Work out the finished part from the listing and answer in its coordinate system (mm). Coordinates: 2 decimals unless noted, no trailing zeros. Write each loop counter-clockwise with the first axis right and the second up, starting at its lowest first coordinate (ties: lowest second). Pieces come first, ordered by that corner, then holes. Notation, with made-up numbers: (43, 16.5) - (91, 16.5) arc R22 ccw to (91, 30.5) - close; hole circle Ø9 at (71.25, 89). An arc over 180 degrees is marked (long way). Answer as a JSON object with one key per item and string values. Group by question number.
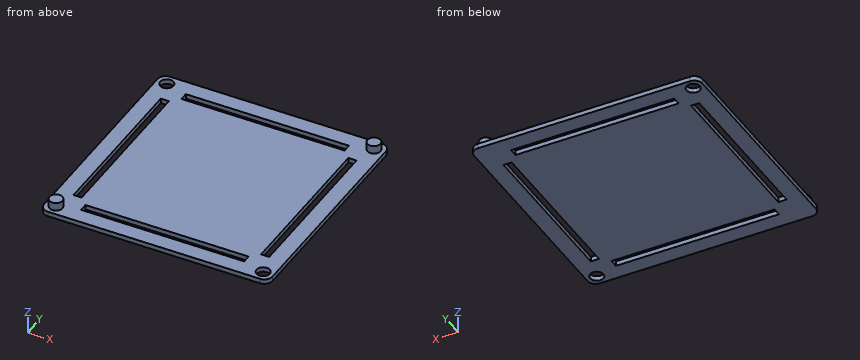
Autodesk Inventor part; units mm, degrees
ref_plane "YZ Plane" through (0, 0, 0) normal (1, 0, 0) x (0, 1, 0)
ref_plane "XZ Plane" through (0, 0, 0) normal (0, 1, 0) x (-1, 0, 0)
ref_plane "XY Plane" through (0, 0, 0) normal (0, 0, 1) x (1, 0, 0)
sketch "Sketch1" plane through (0, 0, 0) normal (0, 0, 1) x (1, 0, 0)
  line L0 (0, 0) -> (140, 0)
  line L1 (140, 0) -> (140, 140)
  line L2 (140, 140) -> (0, 140)
  line L3 (0, 140) -> (0, 0)
  dimension "d0" = 140
  dimension "d1" = 140
extrude "Extrusion1" add sketch "Sketch1" along normal blind 3
fillet "Fillet1" radius 5 4 edges at (140, 140, 1.5) (140, 0, 1.5) (0, 140, 1.5) (0, 0, 1.5)
sketch "Sketch4" plane through (0, 0, 3) normal (0, 0, 1) x (1, 0, 0)
  line L0 (135, 140) -> (5, 140)
  line L1 (0, 135) -> (0, 5)
  line L2 (140, 5) -> (140, 135)
  line L3 (5, 0) -> (135, 0)
  point P0 (0, 0)
  point P1 (6.5, 133.5)
  point P2 (133.5, 6.5)
  dimension "d30" = 6.5
  dimension "d31" = 6.5
  dimension "d34" = 6.5
  dimension "d35" = 6.5
hole "Hole2" at (133.5, 6.5, 3) at (6.5, 133.5, 3) direction (0, 0, -1) diameter 8.2 depth 15
sketch "Sketch5" plane through (0, 0, 3) normal (0, 0, 1) x (1, 0, 0)
  line L0 (20, 130) -> (120, 130)
  line L1 (120, 130) -> (120, 125)
  line L2 (120, 125) -> (20, 125)
  line L3 (20, 125) -> (20, 130)
  line L4 (135, 140) -> (5, 140)
  line L5 (140, 5) -> (140, 135)
  line L6 (20, 15) -> (120, 15)
  line L7 (120, 15) -> (120, 10)
  line L8 (120, 10) -> (20, 10)
  line L9 (20, 10) -> (20, 15)
  line L10 (5, 0) -> (135, 0)
  line L11 (10, 120) -> (15, 120)
  line L12 (15, 120) -> (15, 20)
  line L13 (15, 20) -> (10, 20)
  line L14 (10, 20) -> (10, 120)
  line L15 (0, 135) -> (0, 5)
  line L16 (125, 120) -> (130, 120)
  line L17 (130, 120) -> (130, 20)
  line L18 (130, 20) -> (125, 20)
  line L19 (125, 20) -> (125, 120)
  point P0 (0, 0)
  dimension "d45" = 10
  dimension "d46" = 5
  dimension "d47" = 20
  dimension "d48" = 100
  dimension "d49" = 100
  dimension "d50" = 5
  dimension "d51" = 20
  dimension "d52" = 10
  dimension "d53" = 5
  dimension "d54" = 100
  dimension "d55" = 20
  dimension "d56" = 10
  dimension "d57" = 5
  dimension "d58" = 100
  dimension "d59" = 10
  dimension "d60" = 20
extrude "Extrusion4" cut sketch "Sketch5" against normal blind 10
sketch "Sketch6" plane through (0, 0, 3) normal (0, 0, 1) x (1, 0, 0)
  circle A0 centre (6.5, 6.5) radius 4
  circle A1 centre (133.5, 133.5) radius 4
  line L0 (135, 140) -> (5, 140)
  line L1 (140, 5) -> (140, 135)
  line L2 (5, 0) -> (135, 0)
  line L3 (0, 135) -> (0, 5)
  point P0 (0, 0)
  dimension "d66" = 8
  dimension "d67" = 8
  dimension "d68" = 6.5
  dimension "d69" = 6.5
  dimension "d70" = 6.5
  dimension "d71" = 6.5
extrude "Extrusion5" add sketch "Sketch6" along normal blind 5
properties part number "Led deksel niet hub"
Q1. Section C-C on z = 5.5 is taken. Determine the outline of the cut face in (x, y).
Q2. Section D-D on y = 17 is taken. Determine the outline of the cut face in (x, z).
Q3. Section A-A on x = 53 is taken. Determine the outline of the cut face in (y, z), plus the area to 3 significant figures.
Q4. Consider L1, parallel to X at y = 46, z = 2.25; L2, parallel to Y at x = 6.5, z = 1.25. Determine where each line is inside the solid, lowest interval first. Write a range as from..to.
Q5. Flat-ended cylindrical pins translate along their axes: pin 1 Ø2 at (x, y) = (36.5, 28.5) entering from +Z; pin 2 Ø2 at (y, z) = (101, 5.5) entering from -X. Find the tip coordinate at first contact, or state that the pin passes through.
Numbers:
{
 "1": {"outline": "circle Ø8 at (6.5, 6.5); circle Ø8 at (133.5, 133.5)"},
 "2": {"outline": "(0, 0) - (140, 0) - (140, 3) - (0, 3) - close"},
 "3": {"outline": "(0, 0) - (10, 0) - (10, 3) - (0, 3) - close; (15, 0) - (125, 0) - (125, 3) - (15, 3) - close; (130, 0) - (140, 0) - (140, 3) - (130, 3) - close", "area": "390 mm²"},
 "4": {"L1": "x = 0..10, 15..125, 130..140", "L2": "y = 0..129.4, 137.6..140"},
 "5": {"pin 1": "stops at z = 3", "pin 2": "passes through"}
}
